The model under review builds one solid part; all positions refer to its coordinate system, in mm. Face numbers are marked on the shaded views. A direction names the side the tool comes from. Coordinates: 2 decimals unless noted, no trailing zeros. Order: outer loops, then holes, each group sorted by start corner. A loop starts at its lowest first (then second) coordinate and runs counter-clockwise, first axis right, second up. Notation, with made-up numbers: M 36,-4.5 L 56,-4.5 A18 cw 56,21.5 Z; hole C 57,87.25 d7. An arc over 180 degrees is marked long. Answer as CSV lines item,"result". Start each with the question number.
Q1. Wall thickness on L1, parallel to Y at x = -9.75, z = -8.5; L2, parallel to Z at x = -1.5, y = -23; L3, parallel to Z at x = -14, y = -12: over which ranges is each line inside the solid? List them lowest first. Write a range as [from, to].
Q2. Consider section A-A on x = -21.25. Write out the cut boundary in (y, z), and give its area (3 significant figures).
Q3. Consider section D-D on x = -3. Write out the cut boundary in (y, z).
Q4. For P1, Ø2.5, axis at y = -23, z = -14, coming from the -X side; P2, Ø2, axis at y = -16.5, z = -7.5, coming from the +X side; P3, Ø2, axis at y = 8.5, z = -17, coming from the +X side; P4, Ø10, axis at x = -23, z = -5, coming from the +Y side, all flat-tipped, find the tip position at first contact; note any pin that passes through.
Q5. Consider section B-B on x = -7.25. Write out the cut boundary in (y, z), and give its area (3 significant figures).
Q6. Consider section C-C on y = 2. Write out the cut boundary in (x, z).
Q7. The part is to be moulded in two halves that separate along Z. For the marked faces 3, 4, 5 and 6, say which applies: +Z half, -Z half, draft (parallel to the pull), parting line (faces both ways), or undercut.
Q8. Machinability: for the marked faces 1 and 2, which of the approach directions +Z, -Z, +X, -X, +Y, -Y give a long, thin tool a straight path to every point of the face, cutting with its end or side? Answer none if there is none.
from build123d import *

# Parameters (mm, degrees)
ESQUISSE1_W             = 48
ESQUISSE1_H             = 48
BOSS_EXTRU_1_DEPTH      = 27.2
ESQUISSE1_5_R           = 3.120993446
ENL_V_MAT_EXTRU_1_DEPTH = 24.2
ESQUISSE1_6_R           = 2.1
ENL_V_MAT_EXTRU_2_DEPTH = 6
ESQUISSE1_8_R           = 2.1
ENL_V_MAT_EXTRU_3_DEPTH = 16
BOSS_EXTRU_3_DEPTH      = 4
ESQUISSE1_9_R           = 1
ENL_V_MAT_EXTRU_4_DEPTH = 10
ENL_V_START             = 10
ESQUISSE1_10_R          = 1
ENL_V_MAT_EXTRU_5_DEPTH = 10
CONG_1_R                = 5


with BuildPart() as part:
    # Esquisse1 → Boss.-Extru.1 (new body)
    with BuildSketch(Plane(origin=(0, 0, 0), x_dir=(0, 0, -1), z_dir=(1, 0, 0))):
        with Locations((0, -1)):
            Rectangle(ESQUISSE1_W, ESQUISSE1_H)
    extrude(amount=-BOSS_EXTRU_1_DEPTH)

    # Esquisse1<5> → Enlèv. mat.-Extru.1 (cut)
    # profile 1 of 4: a face of its own
    with BuildSketch(Plane(origin=(0, 0, 0), x_dir=(0, 0, -1), z_dir=(1, 0, 0))):
        with BuildLine():
            ThreePointArc((-14.162038672, 7), (-14.05045442, 5.235939905), (-13.717480384, 3.5))
            ThreePointArc((-13.717480384, 3.5), (-0.162038672, -7), (13.39340304, 3.5))
            ThreePointArc((13.39340304, 3.5), (13.726377076, 5.235939905), (13.837961328, 7))
            Line((13.837961328, 7), (-14.162038672, 7))
        make_face()
    # profile 2 of 4: a face of its own
    with BuildSketch(Plane(origin=(0, 0, 0), x_dir=(0, 0, -1), z_dir=(1, 0, 0))):
        with BuildLine():
            ThreePointArc((13.39340304, 10.5), (8.411175453, 18.067971791), (-0.162038609, 21))
            ThreePointArc((-0.162038609, 21), (-8.735252747, 18.06797183), (-13.717480384, 10.5))
            ThreePointArc((-13.717480384, 10.5), (-14.05045442, 8.764060095), (-14.162038672, 7))
            Line((-14.162038672, 7), (13.837961328, 7))
            ThreePointArc((13.837961328, 7), (13.726377076, 8.764060095), (13.39340304, 10.5))
        make_face()
        with Locations((0, 15)):
            Circle(ESQUISSE1_5_R, mode=Mode.SUBTRACT)
    # profile 3 of 4: a face of its own
    with BuildSketch(Plane(origin=(0, 0, 0), x_dir=(0, 0, -1), z_dir=(1, 0, 0))):
        with BuildLine():
            Line((-14, 3.5), (-14, -21))
            Line((-14, -21), (14, -21))
            Line((14, -21), (14, 3.5))
            Line((14, 3.5), (13.39340304, 3.5))
            ThreePointArc((13.39340304, 3.5), (-0.162038672, -7), (-13.717480384, 3.5))
            Line((-13.717480384, 3.5), (-14, 3.5))
        make_face()
    # profile 4 of 4: a face of its own
    with BuildSketch(Plane(origin=(0, 0, 0), x_dir=(0, 0, -1), z_dir=(1, 0, 0))):
        with Locations((0, 15)):
            Circle(ESQUISSE1_5_R)
    extrude(amount=-ENL_V_MAT_EXTRU_1_DEPTH, mode=Mode.SUBTRACT)

    # Esquisse1<6> → Enlèv. mat.-Extru.2 (cut)
    # profile 1 of 4: a face of its own
    with BuildSketch(Plane(origin=(0, 0, 0), x_dir=(0, 0, -1), z_dir=(1, 0, 0))):
        with BuildLine():
            Line((-17.662038672, 3.5), (-14, 3.5))
            Line((-14, 3.5), (-13.717480384, 3.5))
            ThreePointArc((-13.717480384, 3.5), (-14.05045442, 5.235939905), (-14.162038672, 7))
            ThreePointArc((-14.162038672, 7), (-14.05045442, 8.764060095), (-13.717480384, 10.5))
            Line((-13.717480384, 10.5), (-17.662038672, 10.5))
            ThreePointArc((-17.662038672, 10.5), (-21.162038672, 7), (-17.662038672, 3.5))
        make_face()
        with Locations((-17.662038672, 7)):
            Circle(ESQUISSE1_6_R, mode=Mode.SUBTRACT)
    # profile 2 of 4: a face of its own
    with BuildSketch(Plane(origin=(0, 0, 0), x_dir=(0, 0, -1), z_dir=(1, 0, 0))):
        with Locations((-17.662038672, 7)):
            Circle(ESQUISSE1_6_R)
    # profile 3 of 4: a face of its own
    with BuildSketch(Plane(origin=(0, 0, 0), x_dir=(0, 0, -1), z_dir=(1, 0, 0))):
        with BuildLine():
            Line((13.39340304, 3.5), (14, 3.5))
            Line((14, 3.5), (17.337961328, 3.5))
            ThreePointArc((17.337961328, 3.5), (20.837961328, 7), (17.337961328, 10.5))
            Line((17.337961328, 10.5), (13.39340304, 10.5))
            ThreePointArc((13.39340304, 10.5), (13.726377076, 8.764060095), (13.837961328, 7))
            ThreePointArc((13.837961328, 7), (13.726377076, 5.235939905), (13.39340304, 3.5))
        make_face()
        with Locations((17.337961328, 7)):
            Circle(ESQUISSE1_6_R, mode=Mode.SUBTRACT)
    # profile 4 of 4: a face of its own
    with BuildSketch(Plane(origin=(0, 0, 0), x_dir=(0, 0, -1), z_dir=(1, 0, 0))):
        with Locations((17.337961328, 7)):
            Circle(ESQUISSE1_6_R)
    extrude(amount=-ENL_V_MAT_EXTRU_2_DEPTH, mode=Mode.SUBTRACT)

    # Esquisse1<8> → Enlèv. mat.-Extru.3 (cut)
    with BuildSketch(Plane(origin=(0, 0, 0), x_dir=(0, 0, -1), z_dir=(1, 0, 0))):
        with Locations((-17.662038672, 7)):
            Circle(ESQUISSE1_8_R)
        with Locations((17.337961328, 7)):
            Circle(ESQUISSE1_8_R)
    extrude(amount=-ENL_V_MAT_EXTRU_3_DEPTH, mode=Mode.SUBTRACT)

    # Esquisse2 → Boss.-Extru.3 (add)
    with BuildSketch(Plane.XZ.offset(25)):
        with BuildLine():
            Line((0, 24), (1.906695686, 24))
            ThreePointArc((1.906695686, 24), (0, 0), (1.906695686, -24))
            Line((1.906695686, -24), (0, -24))
            Line((0, -24), (-1.50393066, -24))
            Line((-1.50393066, -24), (-1.50393066, 24))
            Line((-1.50393066, 24), (0, 24))
        make_face()
    extrude(amount=-BOSS_EXTRU_3_DEPTH)

    # Esquisse1<9> → Enlèv. mat.-Extru.4 (cut)
    with BuildSketch(Plane(origin=(0, 0, 0), x_dir=(0, 0, -1), z_dir=(1, 0, 0))):
        with Locations((-14, -23)):
            Circle(ESQUISSE1_9_R)
        with Locations((14, -23)):
            Circle(ESQUISSE1_9_R)
    extrude(amount=-ENL_V_MAT_EXTRU_4_DEPTH, mode=Mode.SUBTRACT)

    # Esquisse1<10> → Enlèv. mat.-Extru.5 (cut)
    with BuildSketch(Plane(origin=(0, 0, 0), x_dir=(0, 0, -1), z_dir=(1, 0, 0)).offset(ENL_V_START)):
        with Locations((-14, -23)):
            Circle(ESQUISSE1_10_R)
        with Locations((14, -23)):
            Circle(ESQUISSE1_10_R)
    extrude(amount=-ENL_V_MAT_EXTRU_5_DEPTH, mode=Mode.SUBTRACT)

    # Congé1
    # the kernel refuses this fillet: 5 mm, written as the material it takes off along each edge
    with BuildSketch(Plane(origin=(-22.2, -20, 19), x_dir=(0, -1, 0), z_dir=(-1, 0, 0))) as cong_1_piece_1_section:
        Polygon((0, 0), (CONG_1_R, 0), (CONG_1_R, CONG_1_R), (0, CONG_1_R), align=None)
    cong_1_piece_1 = extrude(amount=CONG_1_R, mode=Mode.PRIVATE)
    cong_1_piece_1 = cong_1_piece_1 - Plane(origin=(-22.2, -20, 19), x_dir=(0, 0.7071067811865477, -0.7071067811865475), z_dir=(-1, 0, 0)) * Sphere(CONG_1_R, mode=Mode.PRIVATE)
    add(cong_1_piece_1, mode=Mode.SUBTRACT)
    with BuildSketch(Plane(origin=(-22.2, -20, -19), x_dir=(0, -1, 0), z_dir=(-1, 0, 0))) as cong_1_piece_2_section:
        Polygon((0, 0), (CONG_1_R, 0), (CONG_1_R, -CONG_1_R), (0, -CONG_1_R), align=None)
    cong_1_piece_2 = extrude(amount=CONG_1_R, mode=Mode.PRIVATE)
    cong_1_piece_2 = cong_1_piece_2 - Plane(origin=(-22.2, -20, -19), x_dir=(0, 0.7071067811865475, 0.7071067811865476), z_dir=(-1, 0, 0)) * Sphere(CONG_1_R, mode=Mode.PRIVATE)
    add(cong_1_piece_2, mode=Mode.SUBTRACT)
    with BuildSketch(Plane(origin=(-22.2, 18, -19), x_dir=(-1, 0, 0), z_dir=(0, 1, 0))) as cong_1_piece_3_section:
        Polygon((0, 0), (CONG_1_R, 0), (CONG_1_R, -CONG_1_R), (0, -CONG_1_R), align=None)
    cong_1_piece_3 = extrude(amount=CONG_1_R, mode=Mode.PRIVATE)
    cong_1_piece_3 = cong_1_piece_3 - Plane(origin=(-22.2, 18, -19), x_dir=(0.7071067811865475, 0, 0.7071067811865475), z_dir=(0, 1, 0)) * Sphere(CONG_1_R, mode=Mode.PRIVATE)
    add(cong_1_piece_3, mode=Mode.SUBTRACT)
    with BuildSketch(Plane(origin=(-22.2, 18, 19), x_dir=(-1, 0, 0), z_dir=(0, 1, 0))) as cong_1_piece_4_section:
        Polygon((0, 0), (CONG_1_R, 0), (CONG_1_R, CONG_1_R), (0, CONG_1_R), align=None)
    cong_1_piece_4 = extrude(amount=CONG_1_R, mode=Mode.PRIVATE)
    cong_1_piece_4 = cong_1_piece_4 - Plane(origin=(-22.2, 18, 19), x_dir=(0.7071067811865475, 0, -0.7071067811865475), z_dir=(0, 1, 0)) * Sphere(CONG_1_R, mode=Mode.PRIVATE)
    add(cong_1_piece_4, mode=Mode.SUBTRACT)
    with BuildSketch(Plane(origin=(-22.2, -25, 24), x_dir=(0, 0, -1), z_dir=(1, 0, 0)), Plane(origin=(14.406695686, -25, -24), x_dir=(0, 0, 1), z_dir=(-1, 0, 0))) as cong_1_piece_5:
        with BuildLine():
            CenterArc((CONG_1_R, CONG_1_R), CONG_1_R, 180, 90)
            Line((0, CONG_1_R), (0, 0))
            Line((0, 0), (CONG_1_R, 0))
        make_face()
    extrude(amount=36.606695686, mode=Mode.SUBTRACT)
    with BuildSketch(Plane(origin=(-27.2, -25, -19), x_dir=(0, 1, 0), z_dir=(0, 0, 1)), Plane(origin=(-27.2, 18, -24), x_dir=(0, 0, 1), z_dir=(0, -1, 0)), Plane(origin=(-27.2, -20, 24), x_dir=(0, 0, -1), z_dir=(0, 1, 0))) as cong_1_piece_6:
        with BuildLine():
            CenterArc((CONG_1_R, -CONG_1_R), CONG_1_R, 90, 90)
            Line((0, -CONG_1_R), (0, 0))
            Line((0, 0), (CONG_1_R, 0))
        make_face()
    extrude(amount=38, mode=Mode.SUBTRACT)
    with BuildSketch(Plane(origin=(12.5, 23, -24), x_dir=(0, 0, 1), z_dir=(-1, 0, 0))) as cong_1_piece_7:
        with BuildLine():
            CenterArc((CONG_1_R, -CONG_1_R), CONG_1_R, 90, 90)
            Line((0, -CONG_1_R), (0, 0))
            Line((0, 0), (CONG_1_R, 0))
        make_face()
    extrude(amount=34.7, mode=Mode.SUBTRACT)
    with BuildSketch(Plane(origin=(-27.2, 23, 19), x_dir=(1, 0, 0), z_dir=(0, 0, -1))) as cong_1_piece_8:
        with BuildLine():
            CenterArc((CONG_1_R, CONG_1_R), CONG_1_R, 180, 90)
            Line((0, CONG_1_R), (0, 0))
            Line((0, 0), (CONG_1_R, 0))
        make_face()
    extrude(amount=38, mode=Mode.SUBTRACT)
    with BuildSketch(Plane(origin=(12.5, 23, 24), x_dir=(0, 0, -1), z_dir=(-1, 0, 0))) as cong_1_piece_9:
        with BuildLine():
            CenterArc((CONG_1_R, CONG_1_R), CONG_1_R, 180, 90)
            Line((0, CONG_1_R), (0, 0))
            Line((0, 0), (CONG_1_R, 0))
        make_face()
    extrude(amount=34.7, mode=Mode.SUBTRACT)


solid = part.part
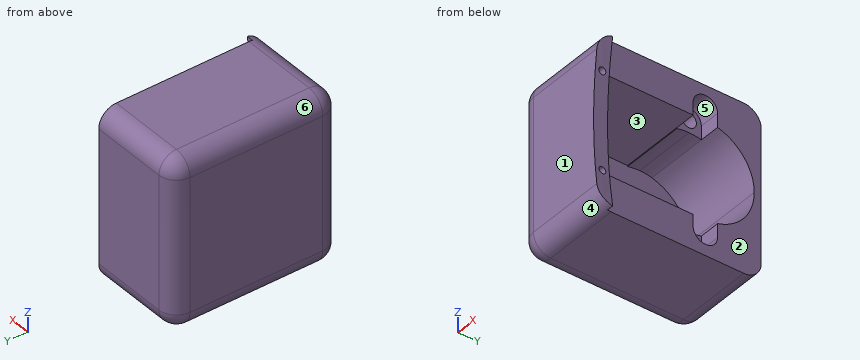
Evaluation:
1,L1,"y = [-25, -21], [18, 23]"
1,L2,"z = [-23, -15], [-13, 13], [15, 23]"
1,L3,"z = [-24, -14], [14, 24]"
2,outline,"M -25,-19 A5 ccw -20,-24 L 18,-24 A5 ccw 23,-19 L 23,19 A5 ccw 18,24 L -20,24 A5 ccw -25,19 Z; hole M -21,-14 L 3.5,-14 L 3.5,-13.39 A14 ccw long 3.5,13.72 L 3.5,14 L -21,14 Z"
2,area,"1,190 mm²"
3,outline,"M -25,-19 A5 ccw -20,-24 L 18,-24 A5 ccw 23,-19 L 23,19 A5 ccw 18,24 L -20,24 A5 ccw -25,19 Z; hole C -23,-14 d2; hole C -23,14 d2; hole M -21,-14 L 3.5,-14 L 3.5,-17.34 A3.5 ccw 10.5,-17.34 L 10.5,-13.39 A14 ccw 10.5,13.72 L 10.5,17.66 A3.5 ccw 3.5,17.66 L 3.5,14 L -21,14 Z"
4,P1,"stops at x = -26.88"
4,P2,"stops at x = -24.2"
4,P3,"stops at x = -6"
4,P4,"stops at y = 23"
5,outline,"M -25,-19 A5 ccw -20,-24 L 18,-24 A5 ccw 23,-19 L 23,19 A5 ccw 18,24 L -20,24 A5 ccw -25,19 Z; hole C -23,-14 d2; hole C -23,14 d2; hole M -21,-14 L 3.5,-14 L 3.5,-13.39 A14 ccw long 3.5,13.72 L 3.5,14 L -21,14 Z; hole C 7,-17.34 d4.2; hole C 7,17.66 d4.2"
5,area,"1,160 mm²"
6,outline,"M -27.2,-19 A5 ccw -22.2,-24 L 0,-24 L 0,-14 L -24.2,-14 L -24.2,14 L 0,14 L 0,24 L -22.2,24 A5 ccw -27.2,19 Z"
7,face 3,"undercut"
7,face 4,"-Z half"
7,face 5,"undercut"
7,face 6,"+Z half"
8,face 1,"+Z, -Z, +X, -X, -Y"
8,face 2,"+Z, -Z, +X, +Y"
